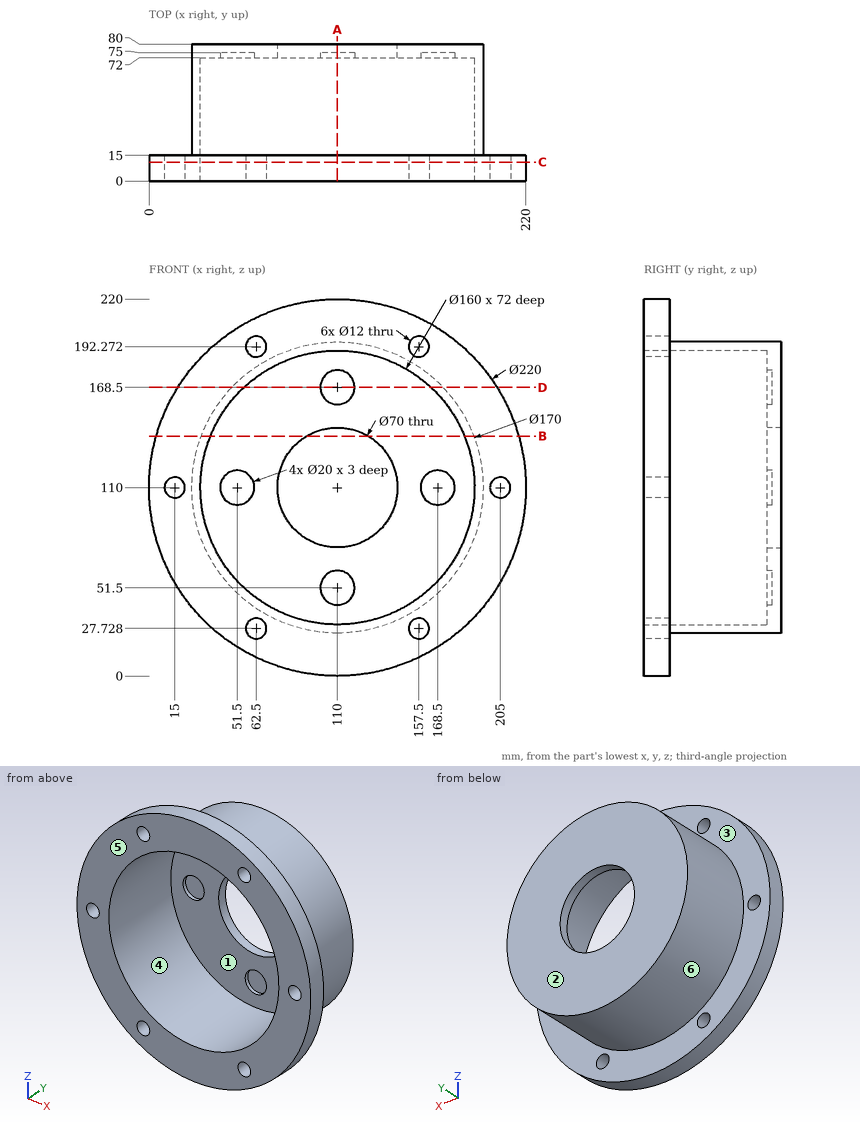
Drawing for the job (mm, zero at the part's lowest x, y, z). A direction names the side the tool comes from. Coordinates: 2 decimals unless noted, no trailing zeros. Order: outer loops, then holes, each group sorted by start corner. A loop starts at its lowest first (then second) coordinate and runs counter-clockwise, first axis right, second up. Notation, with made-up numbers: (-13, -12.75) - (-7, -12.75) arc R17 cw to (-7, 18.25) - close; hole circle Ø2 at (53.5, -16.5). An arc over 180 degrees is marked (long way). Use a Markdown table: item, result. Add a question column.
(1) Drill centre lines: line 1 along X through (y, z) = (74, 110); line 2 along X through (y, z) = (6, 110); line 3 along X through (y, z) = (51, 110). Where is each one in solid material? Low to high. Write a range as [from, to].
(2) Which spindle directions (+Z, -Z, +X, -X, +Y, -Y) get a long thin tool onto all of the face, cutting with end or side? Do the marked faces 1, 2 and 3. Say none if no direction does.
(3) Saw through at C-C (y = 11). Give the cut face in (x, z), then the cut area to 3 significant figures.
(4) Saw through at A-A (x = 110). Give the cut face in (y, z), then the cut area to 3 significant figures.
(5) Saw through at D-D (z = 168.5). Give the cut face in (x, y) (1 decimal).
(6) Saw through at B-B (z = 140). Give the cut face in (x, y), then the cut area to 3 significant figures.
(7) Pull direction X, two halves, no side cores. Call the marked faces 4, 5 and 6: +X half, -X half, draft (parallel to the pull), parting line (faces both ways), or undercut.
(8) Flat gauge pins, fed straight in: pin 1 (1.5 mm diameter, centred on y = 42.5, z = 36.5, fed in from -X); pin 2 (16 mm diameter, centred on x = 106, z = 52, fed in from -Y); pin 3 (5 mm diameter, centred on x = 135.5, y = 38, fed in from +Z). Where does each tip first touch, or does it go through?
Solved:
| question | item | result |
|---|---|---|
| 1 | line 1 | x = [25, 41.5], [61.5, 75], [145, 158.5], [178.5, 195] |
| 1 | line 2 | x = [0, 9], [21, 30], [190, 199], [211, 220] |
| 1 | line 3 | x = [25, 30], [190, 195] |
| 2 | face 1 | -Y |
| 2 | face 2 | +Z, -Z, +X, -X, +Y |
| 2 | face 3 | +Y |
| 3 | outline | circle Ø220 at (110, 110); hole circle Ø12 at (15, 110); hole circle Ø160 at (110, 110); hole circle Ø12 at (62.5, 27.73); hole circle Ø12 at (62.5, 192.27); hole circle Ø12 at (157.5, 27.73); hole circle Ø12 at (157.5, 192.27); hole circle Ø12 at (205, 110) |
| 3 | area | 17,200 mm² |
| 4 | outline | (0, 0) - (15, 0) - (15, 25) - (80, 25) - (80, 75) - (72, 75) - (72, 61.5) - (75, 61.5) - (75, 41.5) - (72, 41.5) - (72, 30) - (0, 30) - close; (0, 190) - (72, 190) - (72, 178.5) - (75, 178.5) - (75, 158.5) - (72, 158.5) - (72, 145) - (80, 145) - (80, 195) - (15, 195) - (15, 220) - (0, 220) - close |
| 4 | area | 2,150 mm² |
| 5 | outline | (16.8, 0) - (55.4, 0) - (55.4, 72) - (100, 72) - (100, 75) - (120, 75) - (120, 72) - (164.6, 72) - (164.6, 0) - (203.2, 0) - (203.2, 15) - (171.7, 15) - (171.7, 80) - (48.3, 80) - (48.3, 15) - (16.8, 15) - close |
| 6 | outline | (4.17, 0) - (35.84, 0) - (35.84, 72) - (91.97, 72) - (91.97, 80) - (30.47, 80) - (30.47, 15) - (4.17, 15) - close; (128.03, 72) - (184.16, 72) - (184.16, 0) - (215.83, 0) - (215.83, 15) - (189.53, 15) - (189.53, 80) - (128.03, 80) - close |
| 6 | area | 2,550 mm² |
| 7 | face 4 | undercut |
| 7 | face 5 | draft |
| 7 | face 6 | parting line |
| 8 | pin 1 | stops at x = 66.04 |
| 8 | pin 2 | stops at y = 72 |
| 8 | pin 3 | stops at z = 191.83 |
